Geometry: see drawing. Coordinates: mm, zero at the bounding-box minimum. A direction names the side the tool comes from. Coordinates: 2 decimals unless noted, no trailing zeros. Loops run counter-clockwise (first coordinate to the right, second up) from the corner with the lowest first, then second, coordinate; pieces in that order, holes last.
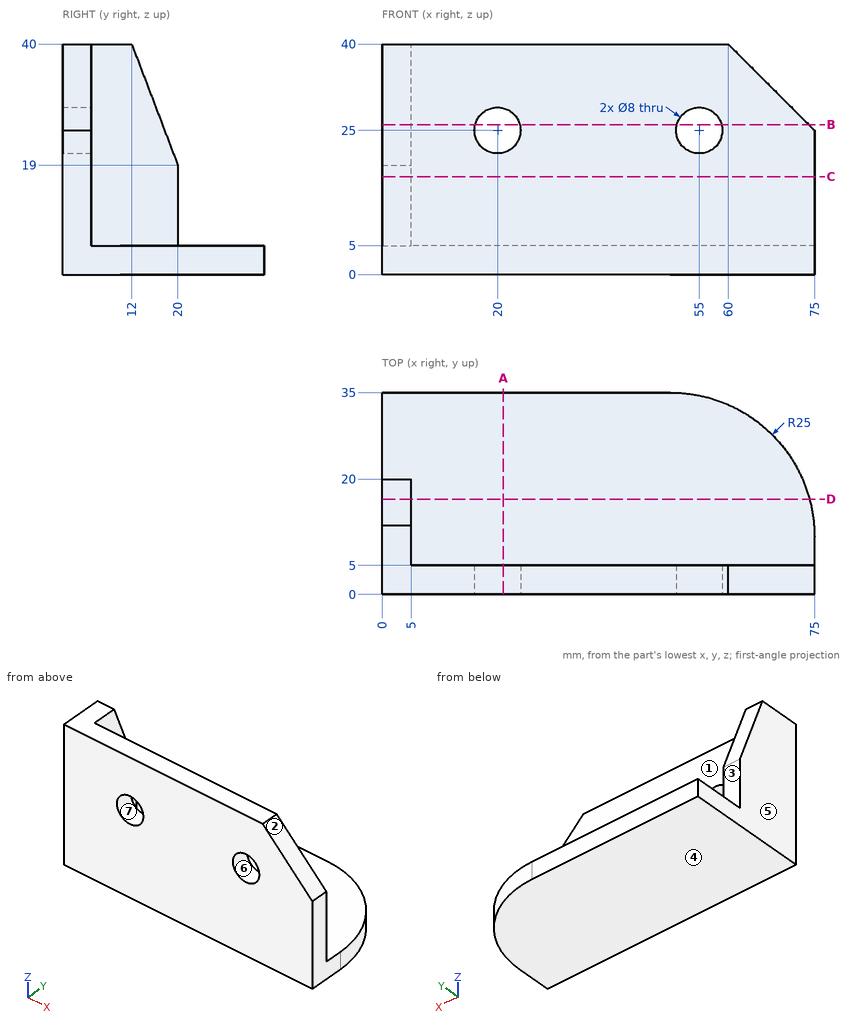
Item 1: Contact query for flat-ended pins moving along their axis: P1, Ø3, axis at x = 22, y = 18.5, coming from the +Z side; P2, Ø2.5, axis at x = 2, z = 13.5, coming from the +Y side; P3, Ø4.5, axis at y = 11, z = 28, coming from the +X side. Output: stop coordinate, or through.
Result:
P1: stops at z = 5
P2: stops at y = 20
P3: stops at x = 5
Item 2: Section query A-A (x = 21). Output: boundary loops of the cut face in (y, z).
Result:
outline: (0, 0) - (35, 0) - (35, 5) - (5, 5) - (5, 21.13) - (0, 21.13) - close; (0, 28.87) - (5, 28.87) - (5, 40) - (0, 40) - close
Item 3: Line query: L1, parallel to X at y = 2.8, z = 25; L2, parallel to Y at x = 40, z = 14.5. Output: solid intervals per line, ascending.
Result:
L1: x = 0 to 16, 24 to 51, 59 to 75
L2: y = 0 to 5
Item 4: Reachability of the marked faces 1, 2 and 3 from +Z, -Z, +X, -X, +Y, -Y: full face, straight path, thin tool, end or side. Return the list, or none.
Result:
face 1: +Z, +X, +Y
face 2: +Z, +X, +Y, -Y
face 3: +Z, +X, -X, +Y
Item 5: Section query D-D (y = 16.5). Output: boundary loops of the cut face in (x, z), then the cut area to 3 significant figures.
Result:
outline: (0, 0) - (74.14, 0) - (74.14, 5) - (5, 5) - (5, 28.19) - (0, 28.19) - close
area: 487 mm2
Item 6: Mould query, pull axis Z, two halves, no side actions, for the marked faces 4, 5, 6 and 7. Classes: +Z half, -Z half, draft (parallel to the pull), parting line (faces both ways), or undercut.
Result:
face 4: -Z half
face 5: draft
face 6: undercut
face 7: undercut
Item 7: Section query C-C (z = 17). Output: boundary loops of the cut face in (x, y).
Result:
outline: (0, 0) - (75, 0) - (75, 5) - (5, 5) - (5, 20) - (0, 20) - close
Item 8: Section query B-B (z = 26). Output: boundary loops of the cut face in (x, y), then the cut area to 3 significant figures.
Result:
outline: (0, 0) - (16.13, 0) - (16.13, 5) - (5, 5) - (5, 17.33) - (0, 17.33) - close; (23.87, 0) - (51.13, 0) - (51.13, 5) - (23.87, 5) - close; (58.87, 0) - (74, 0) - (74, 5) - (58.87, 5) - close
area: 354 mm2
